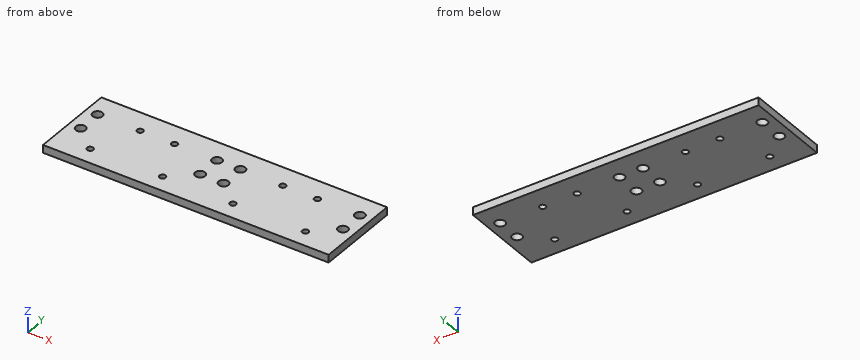
```python
from build123d import *

# Parameters (mm, degrees)
SKETCH1_W           = 116
SKETCH1_H           = 34.5
BOSS_EXTRUDE1_DEPTH = 3.175
SKETCH2_R           = 2
SKETCH2_R_2         = 1.25
CUT_EXTRUDE1_DEPTH  = 95.79098388


with BuildPart() as part:
    # Sketch1 → Boss-Extrude1 (new body)
    with BuildSketch(Plane.XY):
        with Locations((-29, -20.25)):
            Rectangle(SKETCH1_W, SKETCH1_H)
    extrude(amount=BOSS_EXTRUDE1_DEPTH)

    # Sketch2 → Cut-Extrude1 (cut, through all)
    with BuildSketch(Plane(origin=(0, 0, 0), x_dir=(-1, 0, 0), z_dir=(0, 0, -1))):
        with Locations((-24.25, -22.13)):
            Circle(SKETCH2_R)
        with Locations((-24.25, -12.13)):
            Circle(SKETCH2_R)
        with Locations((24.25, -12.13)):
            Circle(SKETCH2_R)
        with Locations((24.25, -22.13)):
            Circle(SKETCH2_R)
        with Locations((33.75, -12.13)):
            Circle(SKETCH2_R)
        with Locations((33.75, -22.13)):
            Circle(SKETCH2_R)
        with Locations((82.25, -12.13)):
            Circle(SKETCH2_R)
        with Locations((82.25, -22.13)):
            Circle(SKETCH2_R)
        with Locations((72.699747468, -30.449747468)):
            Circle(SKETCH2_R_2)
        with Locations((65, -12.13)):
            Circle(SKETCH2_R_2)
        with Locations((51, -12.13)):
            Circle(SKETCH2_R_2)
        with Locations((43.300252532, -30.449747468)):
            Circle(SKETCH2_R_2)
        with Locations((14.699747468, -30.449747468)):
            Circle(SKETCH2_R_2)
        with Locations((7, -12.13)):
            Circle(SKETCH2_R_2)
        with Locations((-7, -12.13)):
            Circle(SKETCH2_R_2)
        with Locations((-14.699747468, -30.449747468)):
            Circle(SKETCH2_R_2)
    extrude(amount=-CUT_EXTRUDE1_DEPTH, mode=Mode.SUBTRACT)


solid = part.part
```
Part model, mm, in its own coordinate system. Give positions to 0.01 mm unless a question says otherwise; leave off trailing zeros. Order: outer loops, then holes, each group sorted by start corner. A loop starts at its lowest first (then second) coordinate and runs counter-clockwise, first axis right, second up. Notation, with made-up numbers: M 62,89 L 104,89 A18 ccw 104,124 Z; hole C 17,10 d1. An arc over 180 degrees is marked long. Use a Markdown table: item, result. Add a question column.
(1) Saw through at C-C, the plane z = 1.9. Give the number of separate pieces and of enclosed holes in the cut face, and give its area (3 significant figures).
(2) Saw through at A-A, the plane x = -65. Give the cut face in (y, z) (3 decimals), and give its area (3 significant figures).
(3) Saw through at B-B, the plane x = -82.25. Give the cut face in (y, z) (3 decimals), and give its area (3 significant figures).
(4) Probe line 1 along Y through (x, z) = (-82.25, 2.5); line 2 along Y through (x, z) = (-51, 2.3); line 3 along X through (y, z) = (-21.5, 0.25). List the from-to ranges inside material, lowest first. Write a range as [from, to].
Answer key:
| question | item | result |
|---|---|---|
| 1 | separate pieces | 1 |
| 1 | enclosed holes | 16 |
| 1 | area | 3,860 mm^2 |
| 2 | outline | M -37.5,0 L -13.38,0 L -13.38,3.175 L -37.5,3.175 Z; M -10.88,0 L -3,0 L -3,3.175 L -10.88,3.175 Z |
| 2 | area | 102 mm^2 |
| 3 | outline | M -37.5,0 L -24.13,0 L -24.13,3.175 L -37.5,3.175 Z; M -20.13,0 L -14.13,0 L -14.13,3.175 L -20.13,3.175 Z; M -10.13,0 L -3,0 L -3,3.175 L -10.13,3.175 Z |
| 3 | area | 84.1 mm^2 |
| 4 | line 1 | [-37.5, -24.13], [-20.13, -14.13], [-10.13, -3] |
| 4 | line 2 | [-37.5, -13.38], [-10.88, -3] |
| 4 | line 3 | [-87, -84.15], [-80.35, -35.65], [-31.85, -26.15], [-22.35, 22.35], [26.15, 29] |
